Work out the finished part from the listing and answer in its coordinate system (mm). Face numbers are marked on the shaded views. A direction names the side the tool comes from. Round coordinates to 2 decimals unless told otherwise and drop trailing zeros. Loops run counter-clockwise (first coordinate to the right, second up) from the corner with the lowest first, then second, coordinate; pieces in that order, holes last. Notation, with made-up numbers: (-29.5, -23.75) -> (5.5, -23.75) arc R19 cw to (5.5, 10.25) -> close; hole circle Ø10 at (10.5, 32.5). An arc over 180 degrees is marked (long way). Write item = value, one per line. Start each with the question number.
```python
from build123d import *

# Parameters (mm, degrees)
F0_R     = 13
F1_DEPTH = 4
F2_SIZE  = 2
F3_R     = 4.7
F4_DEPTH = 3.5
F5_SIZE  = 0.5
F6_R     = 1.5
F7_DEPTH = 25
F8_R     = 5.7
F8_R_2   = 4.7
F9_DEPTH = 1.5


# Not quite as in the source:
# - a fillet or chamfer that OpenCascade refuses, or shapes differently, is made with other operations: its cross-section is extruded or revolved along the edge and cut away or added


with BuildPart() as f1:
    # F0 (on Top) → F1 (new body)
    with BuildSketch(Plane.XY):
        Circle(F0_R)
    extrude(amount=F1_DEPTH)

    # F2
    f2_edges = [f1.edges().sort_by_distance(p)[0] for p in [
        (-13, 0, 4),
    ]]
    chamfer(f2_edges, length=F2_SIZE)

    # F3 (on face) → F4 (join)
    with BuildSketch(Plane(origin=(0, 0, 0), x_dir=(1, 0, 0), z_dir=(0, 0, -1))):
        Circle(F3_R)
    extrude(amount=F4_DEPTH)

    # F5
    f5_edges = [f1.edges().sort_by_distance(p)[0] for p in [
        (-4.7, 0, -3.5),
    ]]
    chamfer(f5_edges, length=F5_SIZE)

    # F6 (on face) → F7 (cut)
    with BuildSketch(Plane(origin=(0, 0, -3.5), x_dir=(1, 0, 0), z_dir=(0, 0, -1))):
        Circle(F6_R)
    extrude(amount=-F7_DEPTH, mode=Mode.SUBTRACT)

    # F8 (on face) → F9 (join)
    with BuildSketch(Plane(origin=(0, 0, 0), x_dir=(1, 0, 0), z_dir=(0, 0, -1))):
        Circle(F8_R)
        Circle(F8_R_2, mode=Mode.SUBTRACT)
    extrude(amount=F9_DEPTH)

    # F10: chamfer of 3 x 8 on 1 edges, made by hand

    # F10_s1 → F10_t2 (revolve, cut)
    with BuildSketch(Plane.XZ):
        Polygon((1.5, 1), (9.5, 4), (1.5, 4), align=None)
    revolve(axis=Axis((0, 0, 4), (0, 0, -1)), mode=Mode.SUBTRACT)


solid = f1.part
```
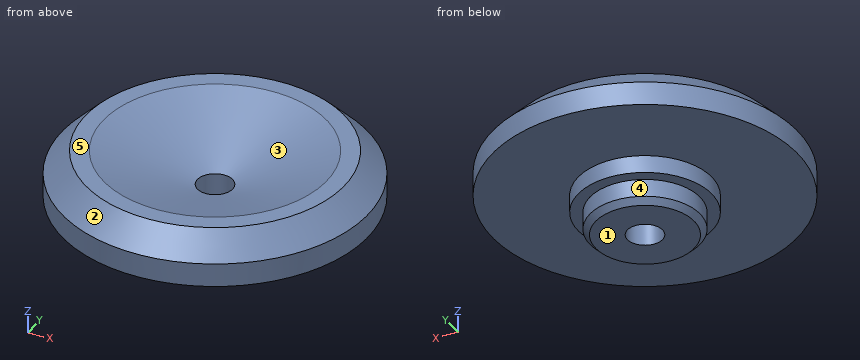
Item 1: Flat-ended cylindrical pins translate along their axes: pin 1 (3 mm diameter, centred on y = 10, z = -0.5, fed in from +X); pin 2 (3 mm diameter, centred on x = -8.5, z = 0, fed in from +Y); pin 3 (1 mm diameter, centred on y = -4, z = 3, fed in from -X). Find the tip coordinate at first contact, or state that the pin passes through.
Item 2: The mould has two halves that part along X. Classify the marked faces 1, 2 and 3: pulls with the +X half, pulls with the -X half, needs draft (parallel to the pull), parting line crosses it, or undercut.
Item 3: A tool of negligible diameter and unlimited length cuts with its end or side. For the marked faces 4 and 5, from which of +Z, -Z, +X, -X, +Y, -Y can it reach the whole face along a straight path? Write none if from no direction.
Item 4: Section C-C (z = 2.5) is taken. Determine the outline of the cut face in (x, y), then the cut area to 3 significant figures.
Item 5: Section A-A (x = 0) is taken. Determine the outline of the cut face in (y, z), then the cut area to 4 significant figures.
Item 6: Find the intervals of material crossed by line 1 along Y through (x, z) = (0, -1.8); line 2 along X through (y, z) = (0, -1.1), in increasing order. Write a range as [from, to].
Worked answers:
q1.pin_1 = 9.76
q1.pin_2 = 10.95
q1.pin_3 = -11.87
q2.face_1 = needs draft
q2.face_2 = parting line crosses it
q2.face_3 = undercut
q3.face_4 = -Z
q3.face_5 = +Z, +X, -X, +Y, -Y
q4.outline = circle Ø25 at (0, 0); hole circle Ø11 at (0, 0)
q4.area = 396 mm2
q5.outline = (-13, 0) -> (-5.7, 0) -> (-5.7, -1.5) -> (-4.7, -1.5) -> (-4.7, -3) -> (-4.2, -3.5) -> (-1.5, -3.5) -> (-1.5, 1) -> (-9.5, 4) -> (-11, 4) -> (-13, 2) -> close; (1.5, -3.5) -> (4.2, -3.5) -> (4.7, -3) -> (4.7, -1.5) -> (5.7, -1.5) -> (5.7, 0) -> (13, 0) -> (13, 2) -> (11, 4) -> (9.5, 4) -> (1.5, 1) -> close
q5.area = 89.15 mm2
q6.line_1 = [-4.7, -1.5], [1.5, 4.7]
q6.line_2 = [-5.7, -1.5], [1.5, 5.7]
